Read the model definition and answer for the solid it produces. Units are mm, in the model's axes. Face numbers are marked on the shaded views. A direction names the side the tool comes from. Round coordinates to 2 decimals unless told otherwise and drop trailing zeros. Loops run counter-clockwise (first coordinate to the right, second up) from the corner with the lowest first, then second, coordinate; pieces in that order, holes last. Notation, with made-up numbers: (87, -19.5) - (93, -19.5) arc R23 cw to (93, 10.5) - close; hole circle Ø4 at (57, 89). An arc over 180 degrees is marked (long way). Use CSV: the item, a comma, the result in double quotes. Start each with the question number.
1. Find section B-B (y = -2.75). Give the vertices of the cut face in (x, z), and give its area (3 significant figures).
2. Consider line 1 along Z through (x, y) = (11.5, -1.5); line 2 along Z through (x, y) = (8.5, -11.25); line 3 along X through (y, z) = (-9.5, -3). Determine where each line is inside the solid, lowest interval first.
3. Given pin 1 Ø4.5 at (x, y) = (5, -11) entering from -Z; pin 2 Ø3 at (x, z) = (1.5, 7) entering from +Y; pin 3 Ø2 at (x, y) = (8, -9.5) entering from -Z, each flat-ended and moving along its own axis, determine where each tip first touches the part or whether it passes through.
4. A tool of negligible diameter and unlimited length cuts with its end or side. For the marked faces 1 and 2, from which of +Z, -Z, +X, -X, +Y, -Y can it reach the whole face along a straight path? Write none if from no direction.
5. Find section C-C (z = -0.75). Give the vertices of the cut face in (x, y), and give its area (3 significant figures).
6. Find section A-A (x = 10.5). Give the vertices of the cut face in (y, z).
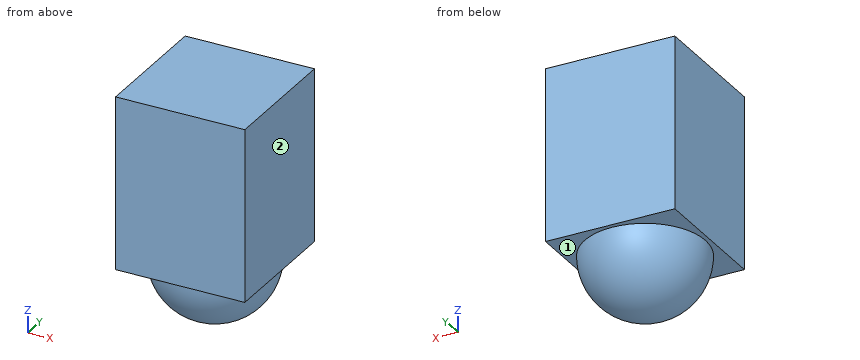
from build123d import *

# Parameters (mm, degrees)
SKETCH1_W           = 15
SKETCH1_H           = 15
BOSS_EXTRUDE1_DEPTH = 20
REVOLVE1_ANGLE      = 180


with BuildPart() as part:
    # Sketch1 → Boss-Extrude1 (new body)
    with BuildSketch(Plane.XY):
        with Locations((7.5, -7.5)):
            Rectangle(SKETCH1_W, SKETCH1_H)
    extrude(amount=BOSS_EXTRUDE1_DEPTH)

    # Sketch2 → Revolve1 (revolve)
    with BuildSketch(Plane(origin=(0, 0, 0), x_dir=(-1, 0, 0), z_dir=(0, 0, -1))):
        with BuildLine():
            Line((-14.5, -7.5), (-0.5, -7.5))
            ThreePointArc((-0.5, -7.5), (-7.5, -14.5), (-14.5, -7.5))
        make_face()
    revolve(axis=Axis((14.5, -7.5, 0), (1, 0, 0)), revolution_arc=REVOLVE1_ANGLE)


solid = part.part
Filled sheet:
1,outline,"(0, 0) - (2.36, 0) arc R5.14 ccw to (12.64, 0) - (15, 0) - (15, 20) - (0, 20) - close"
1,area,"342 mm²"
2,line 1,"z = 0 to 20"
2,line 2,"z = -5.83 to 20"
2,line 3,"x = 1.5 to 13.5"
3,pin 1,"stops at z = -6.69"
3,pin 2,"stops at y = 0"
3,pin 3,"stops at z = -6.92"
4,face 1,"-Z"
4,face 2,"+Z, -Z, +X, +Y, -Y"
5,outline,"circle Ø13.92 at (7.5, -7.5)"
5,area,"152 mm²"
6,outline,"(-15, 0) - (-13.82, 0) arc R6.32 ccw to (-1.18, 0) - (0, 0) - (0, 20) - (-15, 20) - close"
